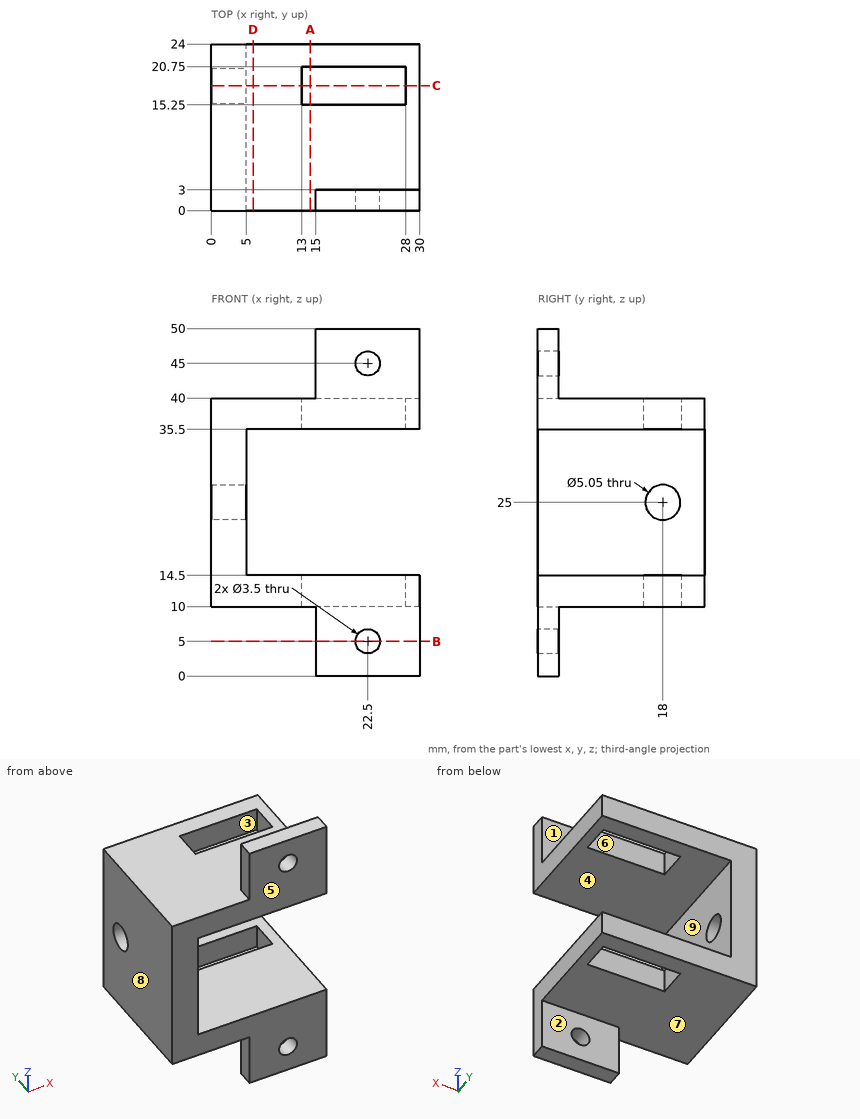
The drawing under review shows one solid part. Ordinate dimensions are in mm from its lowest x, y, z. A direction names the side the tool comes from. Give positions to 0.01 mm unless a question says otherwise; leave off trailing zeros. Order: outer loops, then holes, each group sorted by start corner. A loop starts at its lowest first (then second) coordinate and runs counter-clockwise, first axis right, second up. Notation, with made-up numbers: (27, 41.5) - (64, 41.5) arc R20 cw to (64, 49.5) - close; hole circle Ø3 at (56.25, 41). An arc over 180 degrees is marked (long way). Answer as a JSON object with one key per item and string values. Group by question number.
Item 1: Take a section at D-D on x = 6. Give the boundary of the cut face in (y, z).
Item 2: Wall thickness on line 1 along Z through (x, y) = (10, 5); line 2 along Z through (x, y) = (21, 1.5); line 3 along X through (y, z) = (6.5, 15.5): over which ranges is each line inside the solid? List them lowest first.
Item 3: Take a section at A-A on x = 14.25. Give the boundary of the cut face in (y, z), and give its area (4 significant figures).
Item 4: Clearance check with flat-ended pins moving along their axes: pin 1 Ø6 at (x, y) = (13.5, 15.5) entering from -Z; pin 2 Ø3 at (x, z) = (22, 3.5) entering from +Y. State where each tip first meets the part, or that it passes through.
Item 5: Draft analysis for pull direction X (two halves, no side actions). For the marked faces 6, 7, 8 and 9, state which applies: pulls with the +X half, pulls with the -X half, needs draft (parallel to the pull), parting line crosses it, or undercut.
Item 6: Take a section at B-B on z = 5. Give the boundary of the cut face in (x, y), and give its area (3 significant figures).
Item 7: Take a section at C-C on y = 18. Give the boundary of the cut face in (x, z) (3 decimals).
Item 8: Machinability: for the marked faces 1, 2, 3, 4 and 5, which of the approach directions +Z, -Z, +X, -X, +Y, -Y give a long, thin tool a straight path to every point of the face, cutting with its end or side? Answer none if there is none.
Reported:
{
 "1": {"outline": "(0, 10) - (24, 10) - (24, 14.5) - (0, 14.5) - close; (0, 35.5) - (24, 35.5) - (24, 40) - (0, 40) - close"},
 "2": {"line 1": "10 to 14.5, 35.5 to 40", "line 2": "0 to 4.1, 5.9 to 14.5, 35.5 to 44.1, 45.9 to 50", "line 3": "0 to 5"},
 "3": {"outline": "(0, 10) - (15.25, 10) - (15.25, 14.5) - (0, 14.5) - close; (0, 35.5) - (15.25, 35.5) - (15.25, 40) - (0, 40) - close; (20.75, 10) - (24, 10) - (24, 14.5) - (20.75, 14.5) - close; (20.75, 35.5) - (24, 35.5) - (24, 40) - (20.75, 40) - close", "area": "166.5 mm^2"},
 "4": {"pin 1": "z = 10", "pin 2": "y = 3"},
 "5": {"face 6": "undercut", "face 7": "needs draft", "face 8": "pulls with the -X half", "face 9": "pulls with the +X half"},
 "6": {"outline": "(15, 0) - (20.75, 0) - (20.75, 3) - (15, 3) - close; (24.25, 0) - (30, 0) - (30, 3) - (24.25, 3) - close", "area": "34.5 mm^2"},
 "7": {"outline": "(0, 10) - (13, 10) - (13, 14.5) - (5, 14.5) - (5, 22.475) - (0, 22.475) - close; (0, 27.525) - (5, 27.525) - (5, 35.5) - (13, 35.5) - (13, 40) - (0, 40) - close; (28, 10) - (30, 10) - (30, 14.5) - (28, 14.5) - close; (28, 35.5) - (30, 35.5) - (30, 40) - (28, 40) - close"},
 "8": {"face 1": "+Z, +X, -X, +Y", "face 2": "-Z, +X, -X, +Y", "face 3": "+Z, -Z", "face 4": "+X, +Y, -Y", "face 5": "+Z, -Z, +X, -X, -Y"}
}
